from build123d import *

# Parameters (mm, degrees)
F0_W      = 113.6
F0_H      = 129
F1_DEPTH  = 12.7
F2_W      = 12.7
F2_H      = 129
F3_DEPTH  = 100
F4_R      = 3.175
F5_DEPTH  = 12.7
F6_R      = 5
F7_W      = 12.700058
F7_H      = 129
F8_DEPTH  = 25
F9_W      = 12.6
F9_H      = 85.052852
F10_DEPTH = 12
F11_R     = 5
F12_R     = 3.175
F13_DEPTH = 12.7


with BuildPart() as f1:
    # F0 (on Top) → F1 (new body)
    with BuildSketch(Plane.XY):
        Rectangle(F0_W, F0_H)
    extrude(amount=F1_DEPTH)

    # F2 (on face) → F3 (join)
    with BuildSketch(Plane.XY.offset(12.7)):
        with Locations((-50.45, 0)):
            Rectangle(F2_W, F2_H)
    extrude(amount=F3_DEPTH)

    # F4 (on face) → F5 (cut)
    with BuildSketch(Plane.XZ.offset(64.5)):
        with Locations((-50.45, 96.26574)):
            Circle(F4_R)
    extrude(amount=-F5_DEPTH, mode=Mode.SUBTRACT)

    # F6
    f6_edges = [f1.edges().sort_by_distance(p)[0] for p in [
        (-50.45, -64.5, 112.7),
        (-50.45, 64.5, 112.7),
        (56.8, -64.5, 6.35),
        (56.8, 64.5, 6.35),
    ]]
    fillet(f6_edges, radius=F6_R)

    # F7 (on face) → F8 (join)
    with BuildSketch(Plane(origin=(0, 0, 0), x_dir=(1, 0, 0), z_dir=(0, 0, -1))):
        with Locations((-50.449971, 0)):
            Rectangle(F7_W, F7_H)
    extrude(amount=F8_DEPTH)

    # F9 (on face) → F10 (join)
    with BuildSketch(Plane(origin=(0, 0, 0), x_dir=(1, 0, 0), z_dir=(0, 0, -1))):
        with Locations((6.45, 0)):
            Rectangle(F9_W, F9_H)
    extrude(amount=F10_DEPTH)

    # F11
    f11_edges = [f1.edges().sort_by_distance(p)[0] for p in [
        (0.15, -42.526426, -6),
        (12.75, -42.526426, -6),
        (0.15, 42.526426, -6),
        (12.75, 42.526426, -6),
    ]]
    fillet(f11_edges, radius=F11_R)

    # F12 (on face) → F13 (cut)
    with BuildSketch(Plane(origin=(0, 64.5, 0), x_dir=(-1, 0, 0), z_dir=(0, 1, 0))):
        with Locations((50.45, 96.266)):
            Circle(F12_R)
    extrude(amount=-F13_DEPTH, mode=Mode.SUBTRACT)


solid = f1.part
Check sheet for the modelled part. Datum: model origin and axes. Units: mm. A direction names the side the tool comes from. Give positions to 0.01 mm unless a question says otherwise; leave off trailing zeros. Loops run counter-clockwise (first coordinate to the right, second up) from the corner with the lowest first, then second, coordinate; pieces in that order, holes last. Notation, with made-up numbers: M -5.75,74.25 L 5.25,74.25 A20 ccw 5.25,98.25 Z; hole C 68.25,-28 d4. An arc over 180 degrees is marked long. Return JSON: item names as keys, results as strings. Group by question number.
1. Cross-section at D-D on y = -48. Record the boundary of the cut face in (x, z).
2. Tool access check on faces 4 (the cylindrical face through (1.576, 41.023, -6.084)), 5 (the flat face through (-50, 51.8, 96)), 6 (the cylindrical face through (1.576, -41.023, -6.084)). Record the directions out of +Z, -Z, +X, -X, +Y, -Y that give a thin tool (end or side, any length) a straight path to the whole face; none if there is none.
3. Mould release check, pull along X, two halves, no side actions. Record for faces 1 (the flat face through (6, -1, -12)), 2 (the cylindrical face through (55.3, 63.07, 6.44)), 3 (the flat face through (-44.1, 1, -12)): released by +X, released by -X, zero draft, split by the parting line, or undercut.
4. Thickness scan on L1, parallel to Z at x = -50.45, y = -55.75; L2, parallel to X at y = -3, z = -1.5; L3, parallel to X at y = 16.5, z = 82. Record the ranges inside material, lowest first.
5. Cross-section at A-A on y = -3.5. Record the boundary of the cut face in (x, z).
6. Cross-section at C-C on x = 28. Record the boundary of the cut face in (y, z), plus the area to 3 significant figures.
7. Go/stop test with flat-tipped pins: pin 1 (14 mm diameter, centred on x = 9, y = -0.5, fed in from -Z); pin 2 (0.8 mm diameter, centred on x = 7, z = -7.5, fed in from +Y); pin 3 (3 mm diameter, centred on x = -51, z = 98, fed in from +Y); pin 4 (2 mm diameter, centred on x = 7, z = -3, fed in from -Y). Record where each tip stops, or that it passes through.
8. Cross-section at B-B on z = 63.5. Record the boundary of the cut face in (x, y), plus the area to 3 significant figures.
Return value:
{
 "1": {"outline": "M -56.8,-25 L -44.1,-25 L -44.1,0 L 56.8,0 L 56.8,12.7 L -44.1,12.7 L -44.1,112.7 L -56.8,112.7 Z"},
 "2": {"face 4": "-Z, +Y", "face 5": "+Y", "face 6": "-Z, -Y"},
 "3": {"face 1": "zero draft", "face 2": "released by +X", "face 3": "undercut"},
 "4": {"L1": "-25 to 93.09, 99.44 to 112.7", "L2": "-56.8 to -44.1, 0.15 to 12.75", "L3": "-56.8 to -44.1"},
 "5": {"outline": "M -56.8,-25 L -44.1,-25 L -44.1,0 L 0.15,0 L 0.15,-12 L 12.75,-12 L 12.75,0 L 56.8,0 L 56.8,12.7 L -44.1,12.7 L -44.1,112.7 L -56.8,112.7 Z"},
 "6": {"outline": "M -64.5,0 L 64.5,0 L 64.5,12.7 L -64.5,12.7 Z", "area": "1,640 mm^2"},
 "7": {"pin 1": "z = -12", "pin 2": "y = 42.53", "pin 3": "y = 64.5", "pin 4": "y = -42.53"},
 "8": {"outline": "M -56.8,-64.5 L -44.1,-64.5 L -44.1,64.5 L -56.8,64.5 Z", "area": "1,640 mm^2"}
}
